Source: three-view drawing plus pictorial views. Frame: mm from the lowest corner of the part. A direction names the side the tool comes from. Round coordinates to 2 decimals unless told otherwise and drop trailing zeros. Loops run counter-clockwise (first coordinate to the right, second up) from the corner with the lowest first, then second, coordinate; pieces in that order, holes last. Notation, with made-up numbers: (-2.75, 36.25) -> (39.25, 36.25) arc R17 cw to (39.25, 44.25) -> close; hole circle Ø11 at (42, -31.75). An arc over 180 degrees is marked (long way). Answer in a Markdown table with one row per item. Add a question column.
Q1. Section A-A, the plane z = 27. Output: boundary loops of the cut face in (x, y).
Q2. Ray query, L1, parallel to Y at x = 1.7, z = 27; L2, parallel to Y at x = 40, z = 13; L3, parallel to X at y = 47.5, z = 33. Return the intervals inside material, ascending. Write a range as from..to.
Q3. Reachability of the marked faces 1 and 2 from +Z, -Z, +X, -X, +Y, -Y: full face, straight path, thin tool, end or side. Return the list, or none.
Q4. Section C-C, the plane x = 33.5. Output: boundary loops of the cut face in (y, z).
Q5. Section B-B, the plane y = 28.5. Output: boundary loops of the cut face in (x, z).
Q6. Pin query (flat end, axial travel): pin 1 (4 mm diameter, centred on y = 34.5, z = 73, fed in from +X); pin 2 (10 mm diameter, centred on x = 78, z = 22.5, fed in from +Y); pin 3 (3.5 mm diameter, centred on y = 23.14, z = 27, fed in from -X). Return the tip coordinate at first contact, or that it passes through.
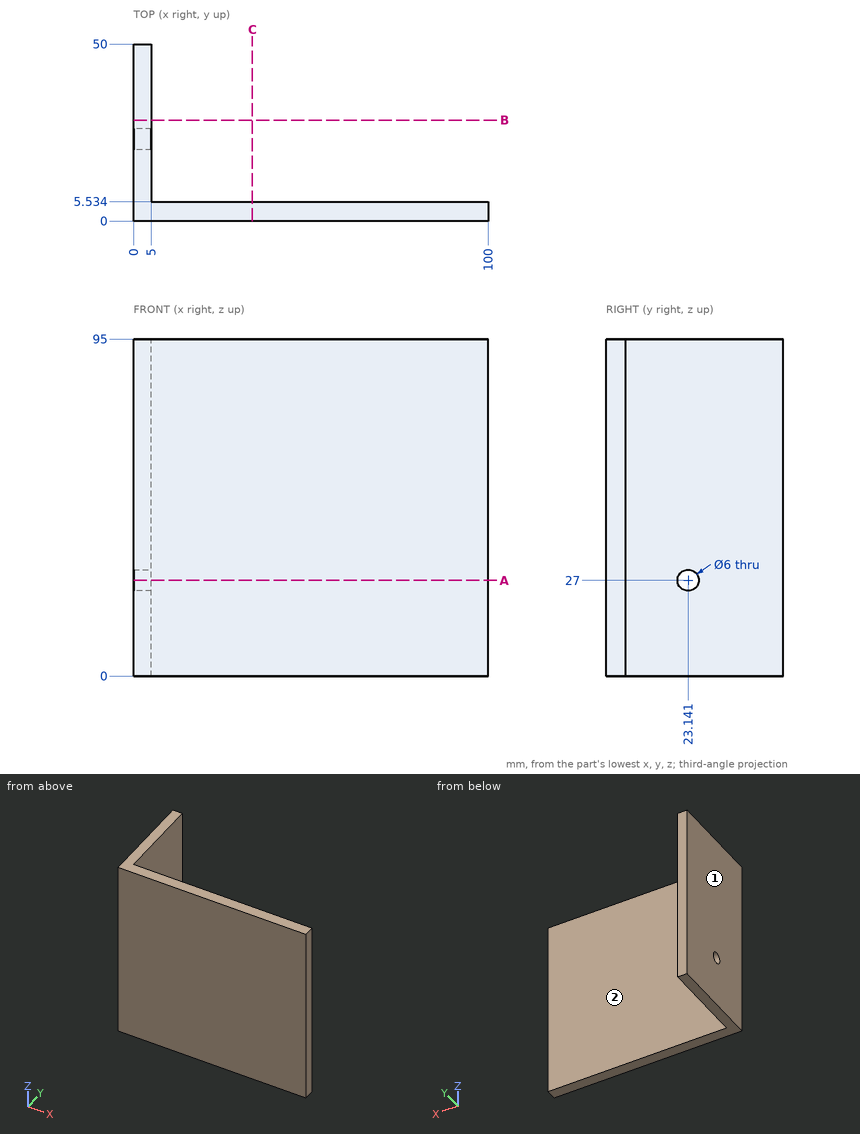
Answer block:
| question | item | result |
|---|---|---|
| 1 | outline | (0, 0) -> (100, 0) -> (100, 5.53) -> (5, 5.53) -> (5, 20.14) -> (0, 20.14) -> close; (0, 26.14) -> (5, 26.14) -> (5, 50) -> (0, 50) -> close |
| 2 | L1 | 0..20.14, 26.14..50 |
| 2 | L2 | 0..5.53 |
| 2 | L3 | 0..5 |
| 3 | face 1 | +Z, -Z, -X, +Y, -Y |
| 3 | face 2 | +Z, -Z, +X, +Y |
| 4 | outline | (0, 0) -> (5.53, 0) -> (5.53, 95) -> (0, 95) -> close |
| 5 | outline | (0, 0) -> (5, 0) -> (5, 95) -> (0, 95) -> close |
| 6 | pin 1 | x = 5 |
| 6 | pin 2 | y = 5.53 |
| 6 | pin 3 | through |
